Geometry check sheet. Reference: the model listing, model coordinates, mm. A direction names the side the tool comes from. Coordinates: 2 decimals unless noted, no trailing zeros. Write each loop counter-clockwise with the first axis right and the second up, starting at its lowest first coordinate (ties: lowest second). Pieces come first, ordered by that corner, then holes. Notation, with made-up numbers: (-22, -13) -> (-13, -13) arc R16 ccw to (-13, 15) -> close; hole circle Ø11 at (0, 80.5). An arc over 180 degrees is marked (long way). One line per question, with ' | ' between items.
Autodesk Inventor part; units mm, degrees
ref_plane "YZ Plane" through (0, 0, 0) normal (1, 0, 0) x (0, 1, 0)
ref_plane "XZ Plane" through (0, 0, 0) normal (0, 1, 0) x (-1, 0, 0)
ref_plane "XY Plane" through (0, 0, 0) normal (0, 0, 1) x (1, 0, 0)
sketch "Sketch1" plane through (0, 0, 0) normal (0, 1, 0) x (-1, 0, 0)
  line L0 (0, 0) -> (-14, 0)
  line L1 (-14, 0) -> (-14, -14)
  line L2 (-14, -14) -> (0, -14)
  line L3 (0, -14) -> (0, 0)
  dimension "d0" = 14
  dimension "d1" = 14
extrude "Extrusion1" add sketch "Sketch1" along normal blind 6
sketch "Sketch2" plane through (0, 0, 0) normal (0, 0, 1) x (1, 0, 0)
  line L0 (0, 0) -> (14, 0)
  line L1 (14, 0) -> (14, 6)
  line L2 (0, 6) -> (14, 6)
  line L3 (0, 0) -> (0, 6)
  line L4 (0.7143, 6) -> (2.2143, 6)
  line L5 (2.2143, 6) -> (2.2143, 1.6)
  line L6 (2.2143, 1.6) -> (0.7143, 1.6)
  line L7 (0.7143, 1.6) -> (0.7143, 6)
  line L8 (0.7143, 3.8) -> (0, 3.8) construction
  line L9 (4.4286, 6) -> (4.4286, 1.6)
  line L10 (4.4286, 1.6) -> (2.9286, 1.6)
  line L11 (2.9286, 1.6) -> (2.9286, 6)
  line L12 (2.9286, 3.8) -> (2.2143, 3.8) construction
  line L13 (6.6429, 6) -> (6.6429, 1.6)
  line L14 (6.6429, 1.6) -> (5.1429, 1.6)
  line L15 (5.1429, 1.6) -> (5.1429, 6)
  line L16 (5.1429, 3.8) -> (4.4286, 3.8) construction
  line L17 (8.8571, 6) -> (8.8571, 1.6)
  line L18 (8.8571, 1.6) -> (7.3571, 1.6)
  line L19 (7.3571, 1.6) -> (7.3571, 6)
  line L20 (7.3571, 3.8) -> (6.6429, 3.8) construction
  line L21 (11.0714, 6) -> (11.0714, 1.6)
  line L22 (11.0714, 1.6) -> (9.5714, 1.6)
  line L23 (9.5714, 1.6) -> (9.5714, 6)
  line L24 (9.5714, 3.8) -> (8.8571, 3.8) construction
  line L25 (0, 6) -> (14, 6)
  line L26 (13.2857, 6) -> (13.2857, 1.6)
  line L27 (13.2857, 1.6) -> (11.7857, 1.6)
  line L28 (11.7857, 1.6) -> (11.7857, 6)
  line L29 (11.7857, 3.8) -> (11.0714, 3.8) construction
  line L30 (13.2857, 3.8) -> (14, 3.8) construction
  dimension "d4" = 6
  dimension "d5" = 1.6
  dimension "d6" = 1.5
  dimension "d8" = 1.5
  dimension "d9" = 1.5
  dimension "d10" = 1.5
  dimension "d11" = 1.5
  dimension "d12" = 1.5
extrude "Extrusion2" cut sketch "Sketch2" against normal through all contours L2 L5 L6 L7 | L26 L27 L28 L2 | L2 L9 L10 L11 | L21 L22 L23 L2 | L2 L13 L14 L15 | L17 L18 L19 L2
properties part number "HEATSINK14x14" material "Aluminum 6061"
(1) Cross-section at A-A (y = 2.05). Record the cut outline in (x, z), plus the area to 3 significant figures.
Answers below:
outline: (0, -14) -> (0.71, -14) -> (0.71, 0) -> (0, 0) -> close; (2.21, -14) -> (2.93, -14) -> (2.93, 0) -> (2.21, 0) -> close; (4.43, -14) -> (5.14, -14) -> (5.14, 0) -> (4.43, 0) -> close; (6.64, -14) -> (7.36, -14) -> (7.36, 0) -> (6.64, 0) -> close; (8.86, -14) -> (9.57, -14) -> (9.57, 0) -> (8.86, 0) -> close; (11.07, -14) -> (11.79, -14) -> (11.79, 0) -> (11.07, 0) -> close; (13.29, -14) -> (14, -14) -> (14, 0) -> (13.29, 0) -> close | area: 70.0 mm²
(2) Material ranges on line 1 (Y direction, x = 3.5, z = -12.5), recorded low to high.
Answers below:
line 1: y = 0 to 1.6
(3) Cross-section at B-B (z = -5.5). Record the cut outline in (x, y).
Answers below:
outline: (0, 0) -> (14, 0) -> (14, 6) -> (13.29, 6) -> (13.29, 1.6) -> (11.79, 1.6) -> (11.79, 6) -> (11.07, 6) -> (11.07, 1.6) -> (9.57, 1.6) -> (9.57, 6) -> (8.86, 6) -> (8.86, 1.6) -> (7.36, 1.6) -> (7.36, 6) -> (6.64, 6) -> (6.64, 1.6) -> (5.14, 1.6) -> (5.14, 6) -> (4.43, 6) -> (4.43, 1.6) -> (2.93, 1.6) -> (2.93, 6) -> (2.21, 6) -> (2.21, 1.6) -> (0.71, 1.6) -> (0.71, 6) -> (0, 6) -> close
(4) Tool access check on faces 4 (the face through (7, 2, 0)), 5 (the face through (11.071, 4, -7)). Record the directions out of +Z, -Z, +X, -X, +Y, -Y that give a thin tool (end or side, any length) a straight path to the whole face; none if there is none.
Answers below:
face 4: +Z, +X, -X, +Y, -Y | face 5: +Z, -Z, +Y
(5) Depth check by flat-ended pin: P1, Ø6, axis at x = 12, z = -8.5, coming from the -Y side; P2, Ø1.2, axis at x = 8, z = -10, coming from the +Y side. Enter the tip coordinate at first touch or a pass-through.
Answers below:
P1: stops at y = 0 | P2: stops at y = 1.6
(6) Cross-section at C-C (x = 7.75). Record the cut outline in (y, z), plus the area to 3 significant figures.
Answers below:
outline: (0, -14) -> (1.6, -14) -> (1.6, 0) -> (0, 0) -> close | area: 22.4 mm²
(7) Draft check along X on faces 1 (the face through (14, 3, -7)), 2 (the face through (7, 2, -14)), 3 (the face through (6, 1.6, -7)). Enter one of: pulls with the +X half, pulls with the -X half, needs draft (parallel to the pull), parting line crosses it, or undercut.
Answers below:
face 1: pulls with the +X half | face 2: needs draft | face 3: undercut
